Can you work these out from the drawing? Everything is in mm from the part's minimum corner. A direction names the side the tool comes from. Round coordinates to 2 decimals unless told otherwise and drop trailing zeros. Loops run counter-clockwise (first coordinate to the right, second up) from the corner with the lowest first, then second, coordinate; pieces in that order, holes last. Notation, with made-up numbers: M 56.5,65.5 L 61.5,65.5 A12 cw 61.5,69.5 Z; hole C -27,63.25 d3. An arc over 180 degrees is marked long. Use a Markdown table: item, result.
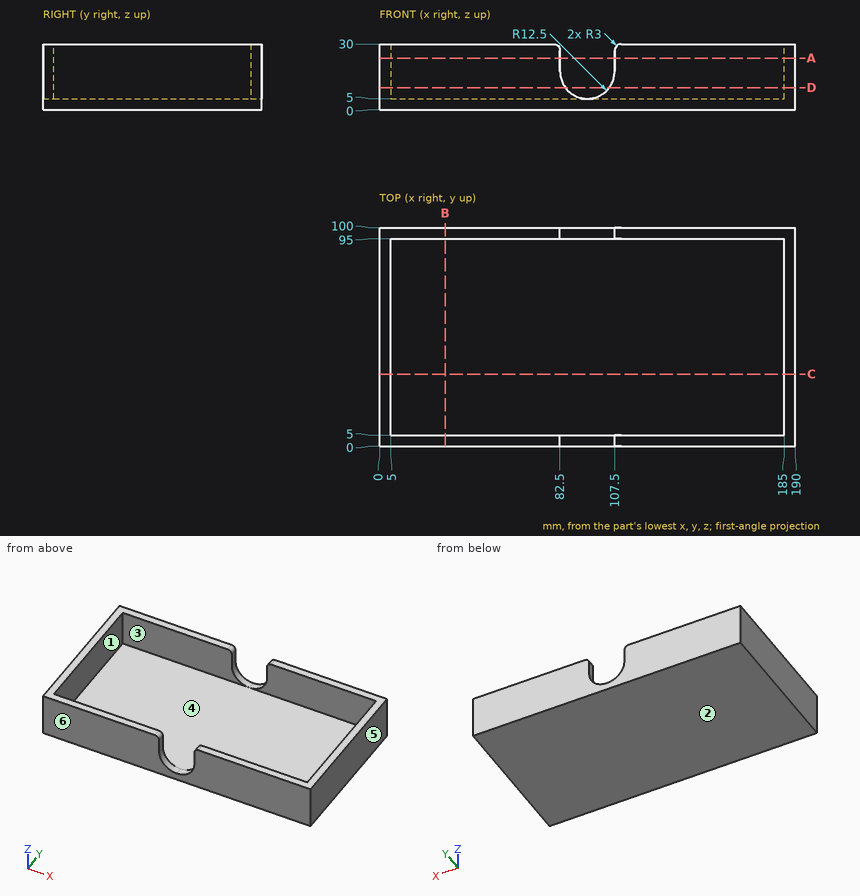
Q1. I need wall thicknesses on line 1 (Y direction, x = 55, z = 6); line 2 (X direction, y = 45, z = 13); line 3 (Z direction, x = 75.5, y = 12.5). Which ranges of each line are inside material? Lowest first, please. Write a range as from..to.
Return value:
| item | result |
|---|---|
| line 1 | y = 0..5, 95..100 |
| line 2 | x = 0..5, 185..190 |
| line 3 | z = 0..5 |
Q2. For the marked faces 1 and 2, which set-ups out of +Z, -Z, +X, -X, +Y, -Y let a thin tool reach every point of the face, with its end or its side?
Return value:
| item | result |
|---|---|
| face 1 | +Z |
| face 2 | -Z, +X, -X, +Y, -Y |
Q3. Imagine slicing it at B-B, the plane x = 30. Please give me the cut outline in (y, z).
Return value:
| item | result |
|---|---|
| outline | M 0,0 L 100,0 L 100,30 L 95,30 L 95,5 L 5,5 L 5,30 L 0,30 Z |
Q4. Imagine slicing it at D-D, the plane z = 10. Please give me the cut outline in (x, y), then the cut area to 3 significant figures.
Return value:
| item | result |
|---|---|
| outline | M 0,0 L 85,0 L 85,5 L 5,5 L 5,95 L 85,95 L 85,100 L 0,100 Z; M 105,0 L 190,0 L 190,100 L 105,100 L 105,95 L 185,95 L 185,5 L 105,5 Z |
| area | 2,600 mm^2 |
Q5. Imagine slicing it at C-C, the plane y = 33. Please give me the cut outline in (x, z).
Return value:
| item | result |
|---|---|
| outline | M 0,0 L 190,0 L 190,30 L 185,30 L 185,5 L 5,5 L 5,30 L 0,30 Z |
Q6. We'd pull the mould along X, two halves only. Please class the marked faces 3, 4, 5 and 6: pulls with the +X half, pulls with the -X half, needs draft (parallel to the pull), parting line crosses it, or undercut.
Return value:
| item | result |
|---|---|
| face 3 | undercut |
| face 4 | undercut |
| face 5 | pulls with the +X half |
| face 6 | needs draft |
Q7. Imagine slicing it at A-A, the plane z = 23.5. Please give me the cut outline in (x, y).
Return value:
| item | result |
|---|---|
| outline | M 0,0 L 82.5,0 L 82.5,5 L 5,5 L 5,95 L 82.5,95 L 82.5,100 L 0,100 Z; M 107.5,0 L 190,0 L 190,100 L 107.5,100 L 107.5,95 L 185,95 L 185,5 L 107.5,5 Z |
